```python
from build123d import *

# Parameters (mm, degrees)
SALIENTE_EXTRUIR1_DEPTH = 10
CORTE_EXTERIOR_R        = 1.5
SALIENTE_EXTRUIR2_DEPTH = 6


with BuildPart() as part:
    # Sketch 0 → Saliente-Extruir1 (new body)
    with BuildSketch(Plane.XY):
        Polygon((35.350833333, 22.415149957), (32.465833333, 22.415149957), (31.023333333, 19.916666667), (32.465833333, 17.418183377), (35.350833333, 17.418183377), (36.793333333, 19.916666667), align=None)
    extrude(amount=SALIENTE_EXTRUIR1_DEPTH)

    # Corte exterior → Saliente-Extruir2 (add)
    with BuildSketch(Plane.XY):
        with Locations((33.908333333, 19.916666667)):
            Circle(CORTE_EXTERIOR_R)
    extrude(amount=-SALIENTE_EXTRUIR2_DEPTH)


solid = part.part
```
Verification items for the finished model (mm, model axes). A direction names the side the tool comes from. Coordinates: 2 decimals unless noted, no trailing zeros. Write each loop counter-clockwise with the first axis right and the second up, starting at its lowest first coordinate (ties: lowest second). Pieces come first, ordered by that corner, then holes. Notation, with made-up numbers: M 78.25,79.5 L 82.25,79.5 A12 ccw 82.25,96.5 Z; hole C 69.5,-34.75 d1. An arc over 180 degrees is marked long. Answer as a JSON object with one key per item and string values. Group by question number.
(1) Cross-section at D-D, the plane z = -1.5. Record the cut outline in (x, y), and give its area (3 significant figures).
(2) Material ranges on line 1 (Z direction, x = 32.1, y = 21.4); line 2 (Y direction, x = 34.6, z = -2.75); line 3 (X direction, y = 18.85, z = -4.5), recorded low to high.
(3) Cross-section at A-A, the plane z = 5.5. Record the cut outline in (x, y), and give its area (3 significant figures).
(4) Tool access check on faces 1 (the face through (35.2, 21.1, 0)), 2 (the face through (36.06, 18.65, 4.93)). Record the directions out of +Z, -Z, +X, -X, +Y, -Y that give a thin tool (end or side, any length) a straight path to the whole face; none if there is none.
(5) Cross-section at B-B, the plane y = 19.4. Record the cut outline in (x, z).
(6) Cross-section at C-C, the plane x = 33.5. Record the cut outline in (y, z).
Reply:
{
 "1": {"outline": "C 33.91,19.92 d3", "area": "7.07 mm²"},
 "2": {"line 1": "0 to 10", "line 2": "18.59 to 21.25", "line 3": "32.85 to 34.96"},
 "3": {"outline": "M 31.02,19.92 L 32.47,17.42 L 35.35,17.42 L 36.79,19.92 L 35.35,22.42 L 32.47,22.42 Z", "area": "21.6 mm²"},
 "4": {"face 1": "-Z", "face 2": "+Z, -Z, +X, -Y"},
 "5": {"outline": "M 31.32,0 L 32.5,0 L 32.5,-6 L 35.32,-6 L 35.32,0 L 36.5,0 L 36.5,10 L 31.32,10 Z"},
 "6": {"outline": "M 17.42,0 L 18.47,0 L 18.47,-6 L 21.36,-6 L 21.36,0 L 22.42,0 L 22.42,10 L 17.42,10 Z"}
}
